For this review, take the finished solid that the model builds, in its own axes (mm). Face numbers are marked on the shaded views. Give positions to 0.01 mm unless a question says otherwise; leave off trailing zeros. Write each loop counter-clockwise with the first axis right and the second up, starting at its lowest first coordinate (ties: lowest second). Pieces come first, ordered by that corner, then holes. Notation, with made-up numbers: M -1.75,33.25 L 6.25,33.25 A9 cw 6.25,45.25 Z; hole C 36,-15.5 d8. An arc over 180 degrees is marked long. Use one line per item in the form item = value. Start each with the question number.
Q1. For probe 1 along Z at (x, y) = (66.5, -63.5); probe 2 along X at (y, z) = (-50.5, 4); probe 3 along X at (y, z) = (-22, 2.25), list the stretches that pass through material, from the lowest coordinate up. Write a range as [from, to].
Q2. Consider section A-A on z = 3. Write out the cut boundary in (x, y), and give its area (3 significant figures).
Q3. Clearance check with flat-ended pins moving along their axes: pin 1 Ø5.5 at (x, y) = (71.55, -8.61) entering from +Z; pin 2 Ø12 at (x, y) = (78.5, -24.5) entering from +Z; pin 3 Ø20 at (x, y) = (70, -46.5) entering from -Z. State where each tip first meets the part, or that it passes through.
Q4. Consider section C-C on x = 69.5. Write out the cut boundary in (y, z), and give its area (3 significant figures).
Q5. Mouldability with a two-part tool opening along Z and no side actions: class the marked faces 1 and 2 as released by +Z, released by -Z, zero draft, split by the parting line, or undercut.
Q6. Consider section B-B on y = -48.5. Write out the cut boundary in (x, z), and give its area (3 significant figures).
Q7. Consider section D-D on y = -8.61. Write out the cut boundary in (x, z).
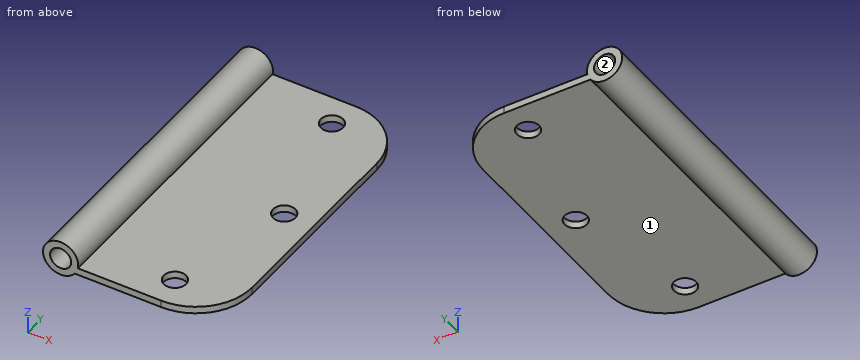
```python
from build123d import *

# Parameters (mm, degrees)
ESQUISSE1_W        = 39.45
ESQUISSE1_H        = 88.646
ESQUISSE1_R        = 3.175
BOSS_EXTRU_1_DEPTH = 2
CONG_1_R           = 15.875
ESQUISSE3_R        = 3
BOSS_EXTRU_2_DEPTH = 88.646


with BuildPart() as part:
    # Esquisse1 → Boss.-Extru.1 (new body)
    with BuildSketch(Plane.XY):
        with Locations((69.175, -44.323)):
            Rectangle(ESQUISSE1_W, ESQUISSE1_H)
        with Locations((80.2894, -44.323)):
            Circle(ESQUISSE1_R, mode=Mode.SUBTRACT)
        with Locations((71.5518, -8.61)):
            Circle(ESQUISSE1_R, mode=Mode.SUBTRACT)
        with Locations(Location((71.5518, -80.036, 0), (0, 0, 180))):
            Circle(ESQUISSE1_R, mode=Mode.SUBTRACT)
    extrude(amount=BOSS_EXTRU_1_DEPTH)

    # Congé1
    cong_1_edges = [part.edges().sort_by_distance(p)[0] for p in [
        (88.9, -88.646, 1),
        (88.9, 0, 1),
    ]]
    fillet(cong_1_edges, radius=CONG_1_R)

    # Esquisse3 → Boss.-Extru.2 (add)
    with BuildSketch(Plane(origin=(0, 0, 0), x_dir=(1, 0, 0), z_dir=(0, 1, 0))):
        with BuildLine():
            Line((49.45, 0), (48.45, 0))
            ThreePointArc((48.45, 0), (39.889522068, -5.049888053), (49.348979486, -2))
            Line((49.348979486, -2), (49.45, -2))
            Line((49.45, -2), (49.45, 0))
        make_face()
        with Locations(Location((44.45, -3, 0), (0, 0, 180))):
            Circle(ESQUISSE3_R, mode=Mode.SUBTRACT)
    extrude(amount=-BOSS_EXTRU_2_DEPTH)


solid = part.part
```
Working result:
q1.probe_1 = [0, 2]
q1.probe_2 = [39.55, 41.62], [47.28, 49.35]
q1.probe_3 = [39.51, 41.55], [47.35, 49.39]
q2.outline = M 39.45,-88.65 L 41.45,-88.65 L 41.45,0 L 39.45,0 Z; M 47.45,-88.65 L 49.45,-88.65 L 49.45,0 L 47.45,0 Z
q2.area = 355 mm²
q3.pin_1 = through
q3.pin_2 = 2
q3.pin_3 = 0
q4.outline = M -88.65,0 L -82.46,0 L -82.46,2 L -88.65,2 Z; M -77.61,0 L -11.03,0 L -11.03,2 L -77.61,2 Z; M -6.19,0 L 0,0 L 0,2 L -6.19,2 Z
q4.area = 158 mm²
q5.face_1 = released by -Z
q5.face_2 = undercut
q6.outline = M 48.45,0 L 88.9,0 L 88.9,2 L 49.35,2 A5 ccw long Z; hole C 44.45,3 d6
q6.area = 130 mm²
q7.outline = M 48.45,0 L 68.38,0 L 68.38,2 L 49.35,2 A5 ccw long Z; M 74.73,0 L 87.14,0 L 87.14,2 L 74.73,2 Z; hole C 44.45,3 d6
